```python
from build123d import *

# Parameters (mm, degrees)
BOSS_EXTRUDE1_DEPTH                        = 100
SKETCH2_R                                  = 2.15
CUT_EXTRUDE1_DEPTH                         = 10
MIRROR1_AT_THE_SECOND_PLANE_COPY_1_SKETC_R = 2.15
MIRROR1_AT_THE_SECOND_PLANE_COPY_1_DEPTH   = 10


with BuildPart() as part:
    # Sketch1 → Boss-Extrude1 (new body)
    with BuildSketch(Plane(origin=(0, 0, 0), x_dir=(1, 0, 0), z_dir=(0, 1, 0))):
        with BuildLine():
            ThreePointArc((31.798147977, -25.07), (0, -40.492309328), (-31.798147977, -25.07))
            Line((-31.798147977, -25.07), (-42.716694629, -25.07))
            ThreePointArc((-42.716694629, -25.07), (0, -49.53), (42.716694629, -25.07))
            Line((42.716694629, -25.07), (31.798147977, -25.07))
        make_face()
    extrude(amount=BOSS_EXTRUDE1_DEPTH)

    # Sketch2 → Cut-Extrude1 (cut)
    with BuildSketch(Plane(origin=(0, 0, 25.07), x_dir=(-1, 0, 0), z_dir=(0, 0, -1))):
        with Locations((-37.257421303, 4.5125)):
            Circle(SKETCH2_R)
    cut_extrude1 = extrude(amount=-CUT_EXTRUDE1_DEPTH, mode=Mode.SUBTRACT)

    # Mirror1: Cut-Extrude1 across plane
    add(cut_extrude1.mirror(Plane(origin=(0, 50, 0), x_dir=(0, 0, 1), z_dir=(0, -1, 0))), mode=Mode.SUBTRACT)

    # Mirror1 at the second plane: Cut-Extrude1 across plane
    add(cut_extrude1.mirror(Plane(origin=(0, 0, 0), x_dir=(0, 0, 1), z_dir=(1, 0, 0))), mode=Mode.SUBTRACT)

    # Mirror1 at the second plane copy 1 sketc → Mirror1 at the second plane copy 1 (cut)
    with BuildSketch(Plane(origin=(0, 100, 25.07), x_dir=(1, 0, 0), z_dir=(0, 0, -1))):
        with Locations((-37.257421303, 4.5125)):
            Circle(MIRROR1_AT_THE_SECOND_PLANE_COPY_1_SKETC_R)
    extrude(amount=-MIRROR1_AT_THE_SECOND_PLANE_COPY_1_DEPTH, mode=Mode.SUBTRACT)


solid = part.part
```
CAD build for the part. Positions are in the model's coordinates, mm. Give positions to 0.01 mm unless a question says otherwise; leave off trailing zeros. Order: outer loops, then holes, each group sorted by start corner. A loop starts at its lowest first (then second) coordinate and runs counter-clockwise, first axis right, second up.
(1) Mould opens along X. For faces 1 (the cylindrical face through (0.51, 49.3, 40.49)), 2 (the cylindrical face through (-0.721, 49.3, 49.525)), 3 (the flat face through (-1, 100, 43)), 4 (the cylindrical face through (35.207, 5.158, 28.839)) say: released by +X, released by -X, zero draft, split by the parting line, or undercut.
(2) Saw through at D-D, the plane x = -26.5. Give the cut face in (y, z).
(3) Flat gauge pins, fed straight in: pin 1 (12 mm diameter, centred on y = 12.5, z = 45, fed in from +X); pin 2 (3 mm diameter, centred on x = 32.5, y = 21.5, fed in from +Z); pin 3 (8 mm diameter, centred on y = 25, z = 31.5, fed in from +X); pin 4 (5.5 mm diameter, centred on x = -37.26, y = 4.51, fed in from -Z). Where does each tip first touch, or does it go through?
(4) Saw through at C-C, the plane y = 30. Give the cut face in (x, z), then the cut area to 3 significant figures.
(5) Saw through at B-B, the plane z = 36.75. Give the cut face in (x, y), then the cut area to 3 significant figures.
(6) Drill centre lines: L1, parallel to X at y = 4, z = 27; L2, parallel to Y at x = -39, z = 28.25; L3, parallel to X at y = 52.5, z = 33.5. Where is each one in solid material? Low to high.
(7) Saw through at A-A, the plane z = 29.5. Give the cut face in (x, y).
Results found:
1. face 1: undercut
1. face 2: split by the parting line
1. face 3: zero draft
1. face 4: undercut
2. outline: (0, 30.62) - (100, 30.62) - (100, 41.84) - (0, 41.84) - close
3. pin 1: stops at x = 30.53
3. pin 2: stops at z = 38.63
3. pin 3: stops at x = 41.19
3. pin 4: stops at z = 25.07
4. outline: (-42.72, 25.07) - (-31.8, 25.07) arc R40.49 cw to (31.8, 25.07) - (42.72, 25.07) arc R49.53 ccw to start
4. area: 797 mm2
5. outline: (-33.21, 0) - (-17, 0) - (-17, 100) - (-33.21, 100) - close; (17, 0) - (33.21, 0) - (33.21, 100) - (17, 100) - close
5. area: 3,240 mm2
6. L1: x = -41.52 to -39.35, -35.17 to -30.18, 30.18 to 35.17, 39.35 to 41.52
6. L2: y = 0 to 3.25, 5.77 to 94.23, 96.75 to 100
6. L3: x = -36.48 to -22.75, 22.75 to 36.48
7. outline: (-39.79, 0) - (-27.74, 0) - (-27.74, 100) - (-39.79, 100) - close; (27.74, 0) - (39.79, 0) - (39.79, 100) - (27.74, 100) - close; hole circle Ø4.3 at (-37.26, 4.51); hole circle Ø4.3 at (-37.26, 95.49); hole circle Ø4.3 at (37.26, 4.51); hole circle Ø4.3 at (37.26, 95.49)
